Can you work these out from the model? Positions are in its coordinate system, mm. A direction names the side the tool comes from. Coordinates: 2 decimals unless noted, no trailing zeros. Order: outer loops, then holes, each group sorted by start corner. A loop starts at its lowest first (then second) coordinate and runs counter-clockwise, first axis right, second up.
Autodesk Inventor part; units mm, degrees
ref_plane "YZ Plane" through (0, 0, 0) normal (1, 0, 0) x (0, 1, 0)
ref_plane "XZ Plane" through (0, 0, 0) normal (0, 1, 0) x (-1, 0, 0)
ref_plane "XY Plane" through (0, 0, 0) normal (0, 0, 1) x (1, 0, 0)
sketch "Esquisse1" plane through (0, 0, 0) normal (1, 0, 0) x (0, 1, 0)
  line L0 (9.85, 20.25) -> (-9.85, 20.25)
  line L1 (-9.85, 20.25) -> (-9.85, -20.25)
  line L2 (-9.85, -20.25) -> (9.85, -20.25)
  line L3 (9.85, -20.25) -> (9.85, 20.25)
  line L4 (9.85, 20.25) -> (-9.85, -20.25)
  line L5 (-9.85, 20.25) -> (9.85, -20.25)
  point P0 (0, 0)
  point P1 (0, 0)
  point P2 (0, 0)
  dimension "d0" = 19.7
  dimension "d1" = 40.5
extrude "Extrusion1" add sketch "Esquisse1" along normal blind 45
sketch "Esquisse2" plane through (0, -9.85, -20.25) normal (0, 0, -1) x (-1, 0, 0)
  line L0 (0, 0) -> (-45, 0)
  line L1 (0, 19.7) -> (-45, 19.7)
  line L2 (-39.8, 0) -> (-37.4, 0)
  line L3 (-37.4, 0) -> (-37.4, 19.7)
  line L4 (-37.4, 19.7) -> (-39.8, 19.7)
  line L5 (-39.8, 19.7) -> (-39.8, 0)
  line L6 (-45, 0) -> (-45, 19.7)
  point P0 (0, 9.85)
  dimension "d4" = 5.2
  dimension "d5" = 2.4
extrude "Extrusion2" add sketch "Esquisse2" along normal blind 7.2 contours L0 L5 L1 L3
sketch "Esquisse3" plane through (0, -9.85, 20.25) normal (0, 0, 1) x (1, 0, 0)
  line L0 (39.8, 19.7) -> (45, 19.7)
  line L1 (39.8, 19.7) -> (37.4, 19.7)
  line L2 (37.4, 19.7) -> (37.4, 0)
  line L3 (37.4, 0) -> (39.8, 0)
  line L4 (39.8, 0) -> (39.8, 19.7)
  point P0 (0, 9.85)
extrude "Extrusion3" add sketch "Esquisse3" along normal blind 7.2
sketch "Esquisse4" plane through (39.8, -9.85, 20.25) normal (1, 0, 0) x (0, 0, -1)
  line L0 (40.5, 19.7) -> (0, 19.7)
  line L1 (20.25, 19.7) -> (20.25, 0)
  line L2 (0, 0) -> (40.5, 0)
  circle A0 centre (-3.6, 14.85) radius 2.25
  line L3 (-7.2, 19.7) -> (-7.2, 0)
  line L4 (-7.2, 9.85) -> (47.7, 9.85)
  line L5 (47.7, 0) -> (47.7, 19.7)
  circle A1 centre (-3.6, 4.85) radius 2.25
  circle A2 centre (44.1, 14.85) radius 2.25
  circle A3 centre (44.1, 4.85) radius 2.25
  point P0 (20.25, 9.85)
  dimension "d10" = 4.5
  dimension "d11" = 10
extrude "Extrusion4" cut sketch "Esquisse4" against normal blind 7.2
sketch "Esquisse5" plane through (45, 0, 0) normal (1, 0, 0) x (0, 0, -1)
  circle A0 centre (-10, 0) radius 6
  point P0 (0, 0)
  dimension "d14" = 12
  dimension "d15" = 10
extrude "Extrusion5" add sketch "Esquisse5" along normal blind 7.2
fillet "Congé1" radius 5 2 edges at (0, 0, 20.25) (0, 0, -20.25)
properties part number "servomoteur_roues"
1. Imagine slicing it at C-C on y = 5. Please give me the cut outline in (x, z).
Completed:
outline: (0, -15.25) arc R5 ccw to (5, -20.25) - (37.4, -20.25) - (37.4, -21.6) - (39.8, -21.6) - (39.8, -20.25) - (45, -20.25) - (45, 6.68) - (52.2, 6.68) - (52.2, 13.32) - (45, 13.32) - (45, 20.25) - (39.8, 20.25) - (39.8, 21.6) - (37.4, 21.6) - (37.4, 20.25) - (5, 20.25) arc R5 ccw to (0, 15.25) - close; (37.4, -27.45) - (39.8, -27.45) - (39.8, -26.1) - (37.4, -26.1) - close; (37.4, 26.1) - (39.8, 26.1) - (39.8, 27.45) - (37.4, 27.45) - close
2. Please list where these lines run through material, in increasing order: probe 1 along Y at (x, z) = (38.8, 23.85); probe 2 along X at (y, z) = (-1.5, 3.5); probe 3 along Z at (x, y) = (41, 8.75).
Completed:
probe 1: y = -9.85 to -7.25, -2.75 to 2.75, 7.25 to 9.85
probe 2: x = 0 to 45
probe 3: z = -20.25 to 20.25
3. On a 3-axis mill with a long thin cutter (end or side, diameter ignored), from which of +Z, -Z, +X, -X, +Y, -Y can I reach the whole of each face in a straight line? I mean faces 1 (the flat face through (42, 0, 20.25)), 2 (the flat face through (37.4, 0, 24)), 3 (the flat face through (37.4, 0, -24)). Say none if no direction works.
Completed:
face 1: +Z, +X, +Y, -Y
face 2: +Z, -X, +Y, -Y
face 3: -Z, -X, +Y, -Y
4. I'm going to push flat-ended pins straight in: pin 1 (6 mm diameter, centred on x = 24, y = 2, fed in from -Z); pin 2 (3 mm diameter, centred on y = -3.5, z = -9.5, fed in from +X); pin 3 (6 mm diameter, centred on y = 2.5, z = -23.5, fed in from +X); pin 4 (4 mm diameter, centred on y = 5, z = -23.85, fed in from +X). Where does each tip first touch, or does it pass through?
Completed:
pin 1: stops at z = -20.25
pin 2: stops at x = 45
pin 3: stops at x = 39.8
pin 4: passes through
5. Imagine slicing it at A-A on z = -23.85. Please give me the cut outline in (x, y), then the cut area to 3 significant figures.
Completed:
outline: (37.4, -9.85) - (39.8, -9.85) - (39.8, -7.25) - (37.4, -7.25) - close; (37.4, -2.75) - (39.8, -2.75) - (39.8, 2.75) - (37.4, 2.75) - close; (37.4, 7.25) - (39.8, 7.25) - (39.8, 9.85) - (37.4, 9.85) - close
area: 25.7 mm2
6. Imagine slicing it at B-B on x = 38.5. Please give me the cut outline in (y, z), then the cut area to 3 significant figures.
Completed:
outline: (-9.85, -27.45) - (9.85, -27.45) - (9.85, 27.45) - (-9.85, 27.45) - close; hole circle Ø4.5 at (-5, -23.85); hole circle Ø4.5 at (-5, 23.85); hole circle Ø4.5 at (5, -23.85); hole circle Ø4.5 at (5, 23.85)
area: 1,020 mm2
7. Imagine slicing it at D-D on y = 8.75. Please give me the cut outline in (x, z).
Completed:
outline: (0, -15.25) arc R5 ccw to (5, -20.25) - (37.4, -20.25) - (37.4, -27.45) - (39.8, -27.45) - (39.8, -20.25) - (45, -20.25) - (45, 20.25) - (39.8, 20.25) - (39.8, 27.45) - (37.4, 27.45) - (37.4, 20.25) - (5, 20.25) arc R5 ccw to (0, 15.25) - close
